Geometry check sheet. Reference: drawing and pictorial views, mm from the part's lowest x, y, z. A direction names the side the tool comes from. Coordinates: 2 decimals unless noted, no trailing zeros. Loops run counter-clockwise (first coordinate to the right, second up) from the corner with the lowest first, then second, coordinate; pieces in that order, holes last. Notation, with made-up numbers: (20, 4) - (36, 4) arc R4 cw to (36, 8) - close; hole circle Ø11 at (70, -37.75). An arc over 180 degrees is marked (long way). Write each question's results on one line, items separated by ' | '. Start each with the question number.
1. Cross-section at D-D (x = 145). Record the cut outline in (y, z).
2. Tool access check on the marked faces 1 and 2. Record the directions out of +Z, -Z, +X, -X, +Y, -Y that give a thin tool (end or side, any length) a straight path to the whole face; none if there is none.
3. Thickness scan on line 1 (Z direction, x = 20, y = 11.8); line 2 (Z direction, x = 154.5, y = 11.75); line 3 (Z direction, x = 51, y = 1). Record the ranges inside material, lowest first. Write a range as [from, to].
4. Gauge pin test, flat ends, axial feed: P1, Ø9, axis at x = 20, z = 30, coming from the +Y side; P2, Ø3, axis at x = 102.5, y = 4, coming from the +Z side; P3, Ø2, axis at x = 114.5, y = 11.5, coming from the +Z side. Record the tip position at first contact, or that the pin passes through.
5. Cross-section at A-A (x = 20). Record the cut outline in (y, z), and give its area (3 significant figures).
6. Cross-section at B-B (z = 22). Record the cut outline in (x, y).
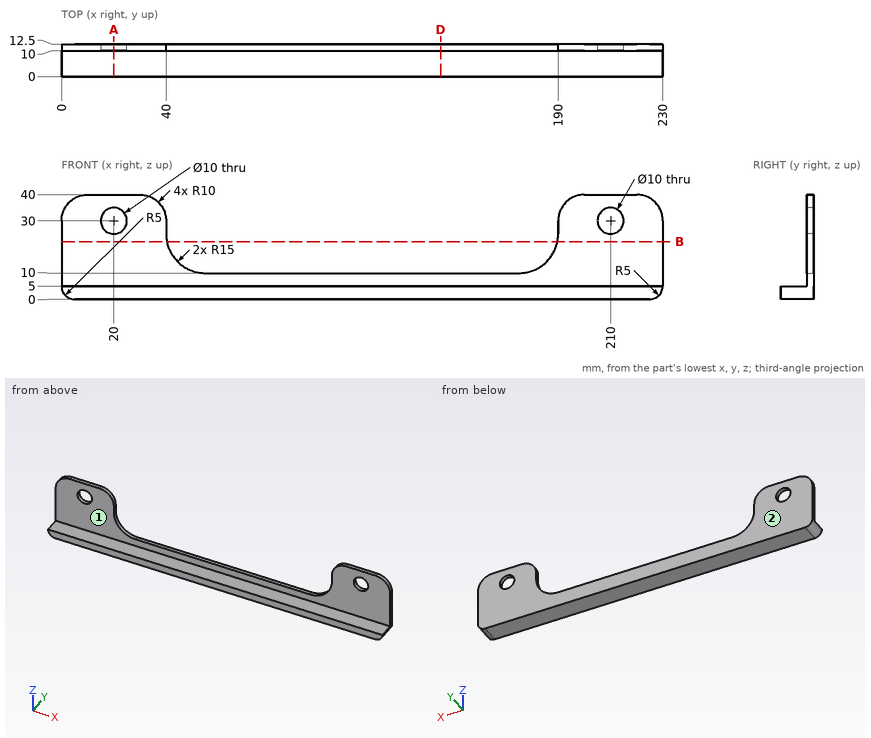
Established:
1) outline: (0, 0) - (12.5, 0) - (12.5, 10) - (10, 10) - (10, 5) - (0, 5) - close
2) face 1: +Z, +X, -X, -Y | face 2: +Z, -Z, +X, -X, +Y
3) line 1: [0, 25], [35, 40] | line 2: [0, 10] | line 3: [0, 5]
4) P1: through | P2: z = 5 | P3: z = 10
5) outline: (0, 0) - (12.5, 0) - (12.5, 25) - (10, 25) - (10, 5) - (0, 5) - close; (10, 35) - (12.5, 35) - (12.5, 40) - (10, 40) - close | area: 125 mm^2
6) outline: (0, 10) - (40.3, 10) - (40.3, 12.5) - (0, 12.5) - close; (189.7, 10) - (230, 10) - (230, 12.5) - (189.7, 12.5) - close
